```python
from build123d import *

# Parameters (mm, degrees)
BOSS_EXTRUDE1_DEPTH = 190.5
SKETCH2_W           = 25.35879418
SKETCH2_H           = 6.35
CUT_EXTRUDE1_DEPTH  = 6.35
LPATTERN1_COUNT     = 3
LPATTERN1_PITCH     = 50.8
BOSS_EXTRUDE2_DEPTH = 6.35
SKETCH5_R           = 2.0955
CUT_EXTRUDE2_DEPTH  = 206.304109574
CUT_EXTRUDE3_DEPTH  = 206.304109574


with BuildPart() as part:
    # Sketch1 → Boss-Extrude1 (new body)
    with BuildSketch(Plane.XY):
        Polygon((-108.212086259, 4.54079067), (-66.902908102, 45.849968827), (-71.393036163, 50.340096887), (-112.702214319, 9.030918731), align=None)
    extrude(amount=BOSS_EXTRUDE1_DEPTH)

    # Sketch2 → Cut-Extrude1 (cut)
    with BuildSketch(Plane(origin=(-60.866566525, 60.866566525, 0), x_dir=(0, 0, 1), z_dir=(-0.7071067811865477, 0.7071067811865474, 0))):
        with Locations((152.42060291, -18.061676125)):
            Rectangle(SKETCH2_W, SKETCH2_H)
        with Locations((152.42060291, -70.131676125)):
            Rectangle(SKETCH2_W, SKETCH2_H)
    cut_extrude1 = extrude(amount=-CUT_EXTRUDE1_DEPTH, mode=Mode.SUBTRACT)

    # LPattern1: Cut-Extrude1 ×3
    with Locations(*[(0, 0, -i * LPATTERN1_PITCH) for i in range(1, LPATTERN1_COUNT)]):
        add(cut_extrude1, mode=Mode.SUBTRACT)

    # Sketch3 → Boss-Extrude2 (add)
    with BuildSketch(Plane(origin=(0, 0, 0), x_dir=(-1, 0, 0), z_dir=(0, 0, -1))):
        Polygon((92.496638047, 20.256238882), (96.986766108, 24.746366942), (88.006509986, 33.726623063), (83.419538791, 29.333338138), align=None)
    extrude(amount=BOSS_EXTRUDE2_DEPTH)

    # Sketch5 → Cut-Extrude2 (cut, through all)
    with BuildSketch(Plane(origin=(-56.376438464, 56.376438464, 0), x_dir=(0, 0, -1), z_dir=(0.7071067811865477, -0.7071067811865474, 0))):
        with Locations(Location((-177.8, -70.131676125, 0), (0, 0, 90))):
            Circle(SKETCH5_R)
        with Locations(Location((-76.2, -70.131676125, 0), (0, 0, 90))):
            Circle(SKETCH5_R)
        with Locations(Location((-15.875, -70.131676125, 0), (0, 0, 90))):
            Circle(SKETCH5_R)
    cut_extrude2 = extrude(amount=-CUT_EXTRUDE2_DEPTH, mode=Mode.SUBTRACT)

    # Mirror1: Cut-Extrude2 across plane
    add(cut_extrude2.mirror(Plane(origin=(-31.181058716, -31.181058716, 0), x_dir=(0, 0, 1), z_dir=(-0.7071067811865475, -0.7071067811865477, 0))), mode=Mode.SUBTRACT)

    # Sketch6 → Cut-Extrude3 (cut, through all)
    with BuildSketch(Plane(origin=(-60.866566525, 60.866566525, 0), x_dir=(0, 0, 1), z_dir=(-0.7071067811865477, 0.7071067811865475, 0))):
        Polygon((52.95420291, -21.236676125), (48.68700291, -21.236676125), (48.68700291, -29.999676125), (46.37560291, -29.999676125), (46.37560291, -33.174676125), (48.68700291, -33.174676125), (48.68700291, -36.476676125), (52.95420291, -36.476676125), (52.95420291, -33.174676125), (55.26560291, -33.174676125), (55.26560291, -29.999676125), (52.95420291, -29.999676125), align=None)
        Polygon((154.55420291, -21.236676125), (150.28700291, -21.236676125), (150.28700291, -29.999676125), (147.97560291, -29.999676125), (147.97560291, -33.174676125), (150.28700291, -33.174676125), (150.28700291, -36.476676125), (154.55420291, -36.476676125), (154.55420291, -33.174676125), (156.86560291, -33.174676125), (156.86560291, -29.999676125), (154.55420291, -29.999676125), align=None)
    cut_extrude3 = extrude(amount=-CUT_EXTRUDE3_DEPTH, mode=Mode.SUBTRACT)

    # Mirror2: Cut-Extrude3 across plane
    add(cut_extrude3.mirror(Plane(origin=(-31.181058716, -31.181058716, 0), x_dir=(0, 0, 1), z_dir=(-0.7071067811865475, -0.7071067811865477, 0))), mode=Mode.SUBTRACT)


solid = part.part
```
Verification items for the finished model (mm, model axes). A direction names the side the tool comes from. Coordinates: 2 decimals unless noted, no trailing zeros. Loops run counter-clockwise (first coordinate to the right, second up) from the corner with the lowest first, then second, coordinate; pieces in that order, holes last. Notation, with made-up numbers: (13.5, 52) -> (48.5, 52) arc R31 ccw to (48.5, 87) -> close; hole circle Ø4 at (80, -39.75). An arc over 180 degrees is marked (long way). Answer in a Markdown table with one row per item. Add a question column.
1. Section check B-B, the plane y = 11. Give the number of separate pieces and of enclosed holes in the cut face, then the cut area to 3 significant figures.
2. Section check A-A, the plane z = 105.5. Enter the section's corners in (x, y).
3. Draft check along X on faces 1 (the face through (-77, 40, 154.554)), 2 (the face through (-85.745, 31.561, -3.131)), 3 (the face through (-70.186, 46.994, 14.6)). Enter one of: +X half, -X half, draft (parallel to the pull), parting line (faces both ways), or undercut.
4. Section check C-C, the plane z = 125.5. Enter the section's corners in (x, y), then the cut area to 3 significant figures.
5. Access from +Z, -Z, +X, -X, +Y, -Y to the whole of each face (thin tool, end or side, straight path). Record for faces 4 (the face through (-73.67, 43.636, 159.753)), 5 (the face through (-108, 9, 38.141)), 6 (the face through (-81, 36, 156.866)).
6. Depth check by flat-ended pin: P1, Ø10, axis at x = -90, z = 37.5, coming from the -Y side; P2, Ø10, axis at y = 21, z = 135, coming from the +X side; P3, Ø1.5, axis at x = -82, y = 32.5, coming from the -Z side. Enter the tip coordinate at first touch or a pass-through.
7. Material ranges on probe 1 along Z at (x, y) = (-78, 41.5); probe 2 along X at (y, z) = (15, 12); probe 3 along X at (y, z) = (36.5, 75.5), recorded low to high. Write a range as [from, to].
Derived:
| question | item | result |
|---|---|---|
| 1 | separate pieces | 3 |
| 1 | enclosed holes | 0 |
| 1 | area | 1,260 mm² |
| 2 | outline | (-108.21, 13.52) -> (-103.72, 9.03) -> (-71.39, 41.36) -> (-75.88, 45.85) -> close |
| 3 | face 1 | draft |
| 3 | face 2 | +X half |
| 3 | face 3 | undercut |
| 4 | outline | (-112.7, 9.03) -> (-108.21, 4.54) -> (-66.9, 45.85) -> (-71.39, 50.34) -> close |
| 4 | area | 371 mm² |
| 5 | face 4 | +X, +Y |
| 5 | face 5 | -X, -Y |
| 5 | face 6 | none |
| 6 | P1 | stops at y = 17.75 |
| 6 | P2 | stops at x = -86.75 |
| 6 | P3 | stops at z = 0 |
| 7 | probe 1 | z = [0, 48.69], [52.95, 150.29], [154.55, 190.5] |
| 7 | probe 2 | x = [-106.73, -97.75] |
| 7 | probe 3 | x = [-85.23, -76.25] |
